```python
from build123d import *

# Parameters (mm, degrees)
SKETCH1_W                = 22
SKETCH1_H                = 14
BOSS_EXTRUDE1_DEPTH      = 14
FILLET1_R                = 2
SKETCH2_R                = 1
CUT_EXTRUDE1_DEPTH       = 19
BOSS_EXTRUDE2_DEPTH      = 3
BOSS_EXTRUDE2_DEPTH_BACK = 31
SKETCH3_W                = 0.554521252
SKETCH3_H                = 9.98669991
SKETCH4_R                = 2
SKETCH4_R_2              = 1.5
BOSS_EXTRUDE3_DEPTH      = 0.8
CUT_EXTRUDE2_START       = -10
SKETCH4_2_R              = 1.5
CUT_EXTRUDE2_DEPTH       = 10
SKETCH5_R                = 7.185985437
BOSS_EXTRUDE5_DEPTH      = 2
BOSS_EXTRUDE6_START      = 2
SKETCH6_R                = 7.341706918
BOSS_EXTRUDE6_DEPTH      = 2
SKETCH7_R                = 1.5
BOSS_EXTRUDE7_DEPTH      = 14
SKETCH8_R                = 1
BOSS_EXTRUDE8_DEPTH      = 14


with BuildPart() as part:
    # Sketch1 → Boss-Extrude1 (new, symmetric)
    with BuildSketch(Plane.XY):
        Rectangle(SKETCH1_W, SKETCH1_H)
    extrude(amount=BOSS_EXTRUDE1_DEPTH, both=True)

    # Fillet1
    fillet1_edges = [part.edges().sort_by_distance(p)[0] for p in [
        (-11, 0, 14),
        (0, -7, 14),
        (11, 0, 14),
        (0, -7, -14),
        (-11, 0, -14),
        (0, 7, -14),
        (11, 0, -14),
        (0, 7, 14),
        (11, -7, 0),
        (-11, -7, 0),
        (-11, 7, 0),
        (11, 7, 0),
    ]]
    fillet(fillet1_edges, radius=FILLET1_R)

    # Sketch2 → Cut-Extrude1 (cut)
    with BuildSketch(Plane.ZY.offset(11)):
        with Locations((-10.565380275, 3.689151377)):
            Circle(SKETCH2_R)
        with Locations((10.5, 3.689151377)):
            Circle(SKETCH2_R)
        with Locations((10.5, -3.4271998)):
            Circle(SKETCH2_R)
        with Locations((-10.565380275, -3.4271998)):
            Circle(SKETCH2_R)
    extrude(amount=-CUT_EXTRUDE1_DEPTH, mode=Mode.SUBTRACT)

    # Sketch3 → Boss-Extrude2 (add, two sides: drawn at the far end of the back side and taken through both)
    with BuildSketch(Plane(origin=(0, 0, -14), x_dir=(-1, 0, 0), z_dir=(0, 0, -1)).offset(-BOSS_EXTRUDE2_DEPTH_BACK)):
        with Locations((-5.504015561, -0.006650045)):
            Rectangle(SKETCH3_W, SKETCH3_H)
    extrude(amount=BOSS_EXTRUDE2_DEPTH + BOSS_EXTRUDE2_DEPTH_BACK)

    # Sketch4 → Boss-Extrude3 (add)
    with BuildSketch(Plane.ZY.offset(11)):
        with Locations(Location((5.416543399, 0, 0), (0, 0, 180))):
            Circle(SKETCH4_R)
        with Locations((5.416543399, 0)):
            Circle(SKETCH4_R_2, mode=Mode.SUBTRACT)
    extrude(amount=BOSS_EXTRUDE3_DEPTH)

    # Sketch4<2> → Cut-Extrude2 (cut)
    with BuildSketch(Plane.ZY.offset(11).offset(CUT_EXTRUDE2_START)):
        with Locations((5.416543399, 0)):
            Circle(SKETCH4_2_R)
    extrude(amount=CUT_EXTRUDE2_DEPTH, mode=Mode.SUBTRACT)

    # Sketch5 → Boss-Extrude5 (add)
    # profile 1 of 2: a face of its own
    with BuildSketch(Plane.XZ.offset(7)):
        with BuildLine():
            Line((2.238059124, 12), (-5.155279816, 17.212901612))
            ThreePointArc((-5.155279816, 17.212901612), (-7.581820377, 17.456866553), (-9.044402043, 15.505335653))
            Line((-9.044402043, 15.505335653), (-9.044402043, 14.86603547))
            Line((-9.044402043, 14.86603547), (-9.044402043, -14.449829967))
            ThreePointArc((-9.044402043, -14.449829967), (-7.529616483, -16.780632089), (-4.78450574, -16.342932608))
            add(Edge.make_bspline(
                [(-4.78450574, -16.342932608), (1.340585112, -14.306096739), (6.77146781, -16.003800215), (11.508142355, -21.436043034)],
                knots=[0.084300371, 0.084300371, 0.084300371, 0.084300371, 1, 1, 1, 1], degree=3))
            ThreePointArc((11.508142355, -21.436043034), (16.041717565, -22.709236327), (18.758055645, -18.862701162))
            Line((18.758055645, -18.862701162), (18.758055645, -1.957446637))
            ThreePointArc((18.758055645, -1.957446637), (18.258122382, 0.092853884), (16.870544719, 1.682914803))
            Line((16.870544719, 1.682914803), (9, 7.232285064))
            Line((9, 7.232285064), (9, -12))
            Line((9, -12), (-9, -12))
            Line((-9, -12), (-9, 12))
            Line((-9, 12), (2.238059124, 12))
        make_face()
    # profile 2 of 2: a face of its own
    with BuildSketch(Plane.XZ.offset(7)):
        Polygon((9, 7.232285064), (2.238059124, 12), (-9, 12), (-9, -12), (9, -12), align=None)
        with Locations(Location((0, 0, 0), (0, 0, 270))):
            Circle(SKETCH5_R, mode=Mode.SUBTRACT)
    extrude(amount=BOSS_EXTRUDE5_DEPTH)

    # Sketch6 → Boss-Extrude6 (add)
    with BuildSketch(Plane(origin=(0, 7, 0), x_dir=(1, 0, 0), z_dir=(0, 1, 0)).offset(BOSS_EXTRUDE6_START)):
        with BuildLine():
            Line((-5.155279816, -17.212901612), (16.870544719, -1.682914803))
            ThreePointArc((16.870544719, -1.682914803), (18.258122382, -0.092853884), (18.758055645, 1.957446637))
            Line((18.758055645, 1.957446637), (18.758055645, 18.862701162))
            ThreePointArc((18.758055645, 18.862701162), (16.041717554, 22.709236331), (11.50814234, 21.436043017))
            add(Edge.make_bspline(
                [(11.50814234, 21.436043017), (4.403130528, 13.287678808), (-4.78450574, 16.342932608)],
                knots=[0, 0, 0, 1, 1, 1], degree=2))
            ThreePointArc((-4.78450574, 16.342932608), (-7.529616483, 16.780632089), (-9.044402043, 14.449829967))
            Line((-9.044402043, 14.449829967), (-9.044402043, -15.505335653))
            ThreePointArc((-9.044402043, -15.505335653), (-7.581820377, -17.456866553), (-5.155279816, -17.212901612))
        make_face()
        with Locations(Location((0, 0, 0), (0, 0, 270))):
            Circle(SKETCH6_R, mode=Mode.SUBTRACT)
    extrude(amount=-BOSS_EXTRUDE6_DEPTH)

    # Sketch7 → Boss-Extrude7 (add)
    with BuildSketch(Plane(origin=(0, -7, 0), x_dir=(1, 0, 0), z_dir=(0, 1, 0))):
        with Locations(Location((14.676397787, 18.862701162, 0), (0, 0, 90))):
            Circle(SKETCH7_R)
    extrude(amount=BOSS_EXTRUDE7_DEPTH)

    # Sketch8 → Boss-Extrude8 (add)
    with BuildSketch(Plane.XZ.offset(-7)):
        with Locations(Location((15.758055645, -1.957446637, 0), (0, 0, 90))):
            Circle(SKETCH8_R)
    extrude(amount=BOSS_EXTRUDE8_DEPTH)


solid = part.part
```
For this review, take the finished solid that the model builds, in its own axes (mm). A direction names the side the tool comes from. Round coordinates to 2 decimals unless told otherwise and drop trailing zeros. Loops run counter-clockwise (first coordinate to the right, second up) from the corner with the lowest first, then second, coordinate; pieces in that order, holes last.
Q1. Mouldability with a two-part tool opening along X and no side actions: class faces 4 (the face through (-7.55, -7.99, 17.47)), 5 (the face through (5.781, -3, 11)), 6 (the face through (-3, -2.6, -10)), 7 (the face through (-4.5, 8, -5.8)) as +X half, -X half, draft (parallel to the pull), parting line (faces both ways), or undercut.
Result sheet:
face 4: parting line
face 5: undercut
face 6: draft
face 7: undercut
Q2. Add section B-B on y = -5.5. Write out the cut boundary in (x, z), plus the area to 3 significant figures.
Result sheet:
outline: (-10.94, -12) arc R1.94 ccw to (-9, -13.94) - (9, -13.94) arc R1.94 ccw to (10.94, -12) - (10.94, 12) arc R1.94 ccw to (9, 13.94) - (-9, 13.94) arc R1.94 ccw to (-10.94, 12) - close; circle Ø3 at (14.68, -18.86); circle Ø2 at (15.76, -1.96)
area: 617 mm2
Q3. Add section C-C on x = -8.5. Write out the cut boundary in (y, z).
Result sheet:
outline: (-9, -16.02) - (-7, -16.02) - (-7, -12) arc R2 ccw to (-5, -14) - (5, -14) arc R2 ccw to (7, -12) - (7, -16.02) - (9, -16.02) - (9, 16.76) - (7, 16.76) - (7, 12) arc R2 ccw to (5, 14) - (-5, 14) arc R2 ccw to (-7, 12) - (-7, 16.76) - (-9, 16.76) - close; hole circle Ø2 at (-3.43, -10.57); hole circle Ø2 at (-3.43, 10.5); hole circle Ø3 at (0, 5.42); hole circle Ø2 at (3.69, -10.57); hole circle Ø2 at (3.69, 10.5)
Q4. Add section A-A on z = -9. Write out the cut boundary in (x, y), plus the area to 3 significant figures.
Result sheet:
outline: (-11, -5) arc R2 ccw to (-9, -7) - (-9.04, -7) - (-9.04, -9) - (18.76, -9) - (18.76, -7) - (9, -7) arc R2 ccw to (11, -5) - (11, 5) arc R2 ccw to (9, 7) - (18.76, 7) - (18.76, 9) - (-9.04, 9) - (-9.04, 7) - (-9, 7) arc R2 ccw to (-11, 5) - close
area: 416 mm2
Q5. To check wall thickness, follow line 1 along Y through (x, z) = (0.5, -13); line 2 along Y through (x, z) = (13, -12); line 3 along X through (y, z) = (-2.25, 9). State the ranges of each line that lie inside material, in increasing order.
Result sheet:
line 1: y = -9 to -7, -6.73 to 6.73, 7 to 9
line 2: y = -9 to -7, 7 to 9
line 3: x = -11 to 11
Q6. Insertion check: pin 1 Ø1.6 at (y, z) = (3.5, 11) entering from -X; pin 2 Ø3 at (y, z) = (-0.5, 4) entering from +X; pin 3 Ø10 at (y, z) = (1.5, -15) entering from +X. Each pin has a flat end and moves straight along its axis. Give the tip position at first contact, or say it passes through.
Result sheet:
pin 1: stops at x = -11
pin 2: stops at x = 11
pin 3: stops at x = 16.18
Q7. Add section D-D on y = 0. Write out the cut boundary in (x, z).
Result sheet:
outline: (-11.8, 3.42) - (-11, 3.42) - (-11, -12) arc R2 ccw to (-9, -14) - (5.23, -14) - (5.23, -17) - (5.78, -17) - (5.78, -14) - (9, -14) arc R2 ccw to (11, -12) - (11, 12) arc R2 ccw to (9, 14) - (5.78, 14) - (5.78, 17) - (5.23, 17) - (5.23, 14) - (-9, 14) arc R2 ccw to (-11, 12) - (-11, 7.42) - (-11.8, 7.42) - (-11.8, 6.92) - (-1, 6.92) - (-1, 3.92) - (-11.8, 3.92) - close; circle Ø3 at (14.68, -18.86); circle Ø2 at (15.76, -1.96)
Q8. Machinability: for faces 1 (the face through (5.781, -3, -11)), 2 (the face through (0, 0, -14)), 3 (the face through (-3, 3.31, -9.64)), which of the approach directions +Z, -Z, +X, -X, +Y, -Y give a long, thin tool a straight path to every point of the face, cutting with its end or side? Answer none if there is none.
Result sheet:
face 1: none
face 2: -Z
face 3: -X
